Autodesk Inventor part; units mm, degrees
ref_plane "YZ Plane" through (0, 0, 0) normal (1, 0, 0) x (0, 1, 0)
ref_plane "XZ Plane" through (0, 0, 0) normal (0, 1, 0) x (-1, 0, 0)
ref_plane "XY Plane" through (0, 0, 0) normal (0, 0, 1) x (1, 0, 0)
sketch "Sketch1" plane through (0, 0, 0) normal (0, 0, 1) x (1, 0, 0)
  line L0 (-1.9536, 0.6855) -> (4.3964, 0.6855)
  line L1 (4.3964, -2.9551) -> (-1.9315, -6.6341)
  line L2 (-1.9315, -6.6341) -> (-8.2815, -2.9935)
  line L3 (-8.2815, -2.9935) -> (-8.3036, 4.3261)
  line L4 (-8.3036, 4.3261) -> (-1.9757, 8.0051)
  line L5 (-1.9757, 8.0051) -> (4.3743, 4.3644)
  line L6 (4.3743, 4.3644) -> (4.3964, -2.9551)
  dimension "d0" = 6.35
extrude "Extrusion1" add sketch "Sketch1" along normal blind 127
properties part number "Hex Shaft"
Verification items for the finished model (mm, model axes). Coordinates: 2 decimals unless noted, no trailing zeros. Order: outer loops, then holes, each group sorted by start corner. A loop starts at its lowest first (then second) coordinate and runs counter-clockwise, first axis right, second up. Notation, with made-up numbers: M -6.75,63 L 45.25,63 A36 cw 45.25,100 Z; hole C -10,-15.5 d4. An arc over 180 degrees is marked long. One line per item, written item: value. Start each with the question number.
Item 1: Depth check by flat-ended pin: P1, Ø3, axis at y = 0.5, z = 95, coming from the +X side; P2, Ø1, axis at y = -5, z = 36.5, coming from the +X side; P3, Ø3, axis at x = -7, z = 42, coming from the +Y side. Enter the tip coordinate at first touch or a pass-through.
Item 2: Sectioned sample at B-B on x = 1. Record the cut outline in (y, z), then the cut area to 3 significant figures.
Item 3: Sectioned sample at A-A on z = 84. Record the cut outline in (x, y), then the cut area to 3 significant figures.
Item 4: Sectioned sample at C-C on x = -4.5. Record the cut outline in (y, z), then the cut area to 3 significant figures.
Item 5: Thickness scan on probe 1 along X at (y, z) = (0.75, 99); probe 2 along Y at (x, z) = (-1, 71); probe 3 along Y at (x, z) = (0.25, 66.5). Record the ranges inside material, lowest first.
Calculated:
1. P1: x = 4.39
1. P2: x = 1.74
1. P3: y = 5.96
2. outline: M -4.93,0 L 6.3,0 L 6.3,127 L -4.93,127 Z
2. area: 1,430 mm^2
3. outline: M -8.3,4.33 L -8.28,-2.99 L -1.93,-6.63 L 4.4,-2.96 L 4.37,4.36 L -1.98,8.01 Z
3. area: 139 mm^2
4. outline: M -5.16,0 L 6.54,0 L 6.54,127 L -5.16,127 Z
4. area: 1,490 mm^2
5. probe 1: -8.29 to 4.39
5. probe 2: -6.09 to 7.45
5. probe 3: -5.37 to 6.73
